Here's how the part is built. I have some questions about the finished solid (model axes, mm). Round coordinates to 2 decimals unless told otherwise and drop trailing zeros. Order: outer loops, then holes, each group sorted by start corner. A loop starts at its lowest first (then second) coordinate and runs counter-clockwise, first axis right, second up. Notation, with made-up numbers: (58.5, -14) - (85.5, -14) arc R19 ccw to (85.5, 12) - close; hole circle Ø6 at (5.5, -20). An arc over 180 degrees is marked (long way). Answer as a JSON object with one key per item and string values.
```python
from build123d import *

# Parameters (mm, degrees)
SKETCH1_W           = 1066.8
SKETCH1_H           = 558.8
BOSS_EXTRUDE1_DEPTH = 3.175
CUT_EXTRUDE1_REACH  = 5.175


with BuildPart() as part:
    # Sketch1 → Boss-Extrude1 (new body)
    with BuildSketch(Plane.XY):
        Rectangle(SKETCH1_W, SKETCH1_H)
    extrude(amount=BOSS_EXTRUDE1_DEPTH)

    # Sketch2 → Cut-Extrude1 (cut, up to next)
    with BuildSketch(Plane.XY.offset(3.175), mode=Mode.PRIVATE) as cut_extrude1_sk1:
        with BuildLine():
            Line((-273.84375, 84.1375), (273.84375, 84.1375))
            ThreePointArc((273.84375, 84.1375), (282.824006121, 80.417756121), (286.54375, 71.4375))
            Line((286.54375, 71.4375), (286.54375, -173.0375))
            ThreePointArc((286.54375, -173.0375), (282.824006121, -182.017756121), (273.84375, -185.7375))
            Line((273.84375, -185.7375), (-273.84375, -185.7375))
            ThreePointArc((-273.84375, -185.7375), (-282.824006121, -182.017756121), (-286.54375, -173.0375))
            Line((-286.54375, -173.0375), (-286.54375, 71.4375))
            ThreePointArc((-286.54375, 71.4375), (-282.824006121, 80.417756121), (-273.84375, 84.1375))
        make_face()
    cut_extrude1_tool1 = extrude(cut_extrude1_sk1.sketch, amount=-CUT_EXTRUDE1_REACH, mode=Mode.PRIVATE) & part.part
    add(cut_extrude1_tool1.solids().sort_by_distance((0, -50.8, 3.175))[0], mode=Mode.SUBTRACT)


solid = part.part
```
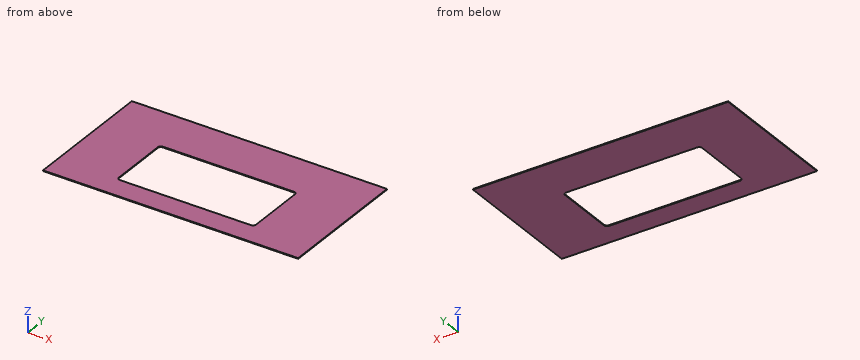
1. Imagine slicing it at B-B (z = 2.3). List the corners of the cut face in (x, y) for me.
Responses:
{"outline": "(-533.4, -279.4) - (533.4, -279.4) - (533.4, 279.4) - (-533.4, 279.4) - close; hole (-286.54, -173.04) arc R12.7 ccw to (-273.84, -185.74) - (273.84, -185.74) arc R12.7 ccw to (286.54, -173.04) - (286.54, 71.44) arc R12.7 ccw to (273.84, 84.14) - (-273.84, 84.14) arc R12.7 ccw to (-286.54, 71.44) - close"}
2. Imagine slicing it at C-C (x = -53). List the corners of the cut face in (y, z) for me (1 decimal), plus the area to 3 significant figures.
Responses:
{"outline": "(-279.4, 0) - (-185.7, 0) - (-185.7, 3.2) - (-279.4, 3.2) - close; (84.1, 0) - (279.4, 0) - (279.4, 3.2) - (84.1, 3.2) - close", "area": "917 mm2"}
3. If I drill on L1, parallel to X at y = -102, z = 1.75; L2, parallel to Y at x = -139, z = 1.8; L3, parallel to Y at x = 283, z = 0.95, over which ranges is the centre line in solid material (lowest first)? Write a range as [from, to].
Responses:
{"L1": "[-533.4, -286.54], [286.54, 533.4]", "L2": "[-279.4, -185.74], [84.14, 279.4]", "L3": "[-279.4, -181.84], [80.24, 279.4]"}
4. Imagine slicing it at A-A (y = 25.5). List the corners of the cut face in (x, z) for me (3 decimals), plus the area to 3 significant figures.
Responses:
{"outline": "(-533.4, 0) - (-286.544, 0) - (-286.544, 3.175) - (-533.4, 3.175) - close; (286.544, 0) - (533.4, 0) - (533.4, 3.175) - (286.544, 3.175) - close", "area": "1,570 mm2"}
